Build history of the part. All positions in model axes, mm. A direction names the side the tool comes from. Give positions to 0.01 mm unless a question says otherwise; leave off trailing zeros. Order: outer loops, then holes, each group sorted by start corner. A loop starts at its lowest first (then second) coordinate and runs counter-clockwise, first axis right, second up. Notation, with made-up numbers: M -0.75,48.5 L 39.25,48.5 A16 ccw 39.25,52.5 Z; hole C -29,56 d5. An arc over 180 degrees is marked long. One line per item, written item: value. Start each with the question number.
Autodesk Inventor part; units mm, degrees
ref_plane "YZ Plane" through (0, 0, 0) normal (1, 0, 0) x (0, 1, 0)
ref_plane "XZ Plane" through (0, 0, 0) normal (0, 1, 0) x (-1, 0, 0)
ref_plane "XY Plane" through (0, 0, 0) normal (0, 0, 1) x (1, 0, 0)
sketch "Sketch1" plane through (0, 0, 0) normal (0, 0, 1) x (1, 0, 0)
  line L0 (0, 0) -> (25.4, 0)
  line L1 (25.4, 0) -> (25.4, 25.4)
  line L2 (25.4, 25.4) -> (0, 25.4)
  line L3 (0, 25.4) -> (0, 0)
  line L4 (1.5875, 23.8125) -> (23.8125, 23.8125)
  line L5 (23.8125, 23.8125) -> (23.8125, 1.5875)
  line L6 (23.8125, 1.5875) -> (1.5875, 1.5875)
  line L7 (1.5875, 1.5875) -> (1.5875, 23.8125)
  dimension "d0" = 25.4
  dimension "d1" = 25.4
  dimension "d2" = 1.5875
extrude "Extrusion1" add sketch "Sketch1" against normal blind 330.2
sketch "Sketch2" plane through (0, 0, 0) normal (0, -1, 0) x (1, 0, 0)
  line L0 (0, -330.2) -> (25.4, -330.2)
  point P0 (12.7, -127)
  point P1 (12.7, -88.9)
  dimension "d5" = 38.1
  dimension "d6" = 203.2
hole "Hole1" at (12.7, 0, -127) at (12.7, 0, -88.9) direction (0, 1, 0) diameter 6.35 depth 25.4 tip angle 118
properties part number "1tube_13_layer1_side"
1) Drill centre lines: line 1 (Z direction, x = 12.7, y = 0.7) (3 decimals); line 2 (X direction, y = 24.35, z = -127) (3 decimals); line 3 (X direction, y = 7.75, z = -239.5). Where is each one in solid material? Low to high.
2) Slice it at B-B (x = 12.7). List the corners of the cut face in (y, z) (1 decimal), plus the area to 3 significant figures.
3) Tool access for faces 1 (the cylindrical face through (13.92, 24.62, -129.93)), 2 (the flat face through (23.812, 13, -163)): list every direction of +Z, -Z, +X, -X, +Y, -Y with a clear straight run to the whole face (end or side of a thin tool).
4) Pull direction Y, two halves, no side cores. Call faces 3 (the flat face through (13, 25.4, -163)), 4 (the flat face through (13, 1.588, -163)), 5 (the cylindrical face through (13.92, 0.8, -129.93)): pulls with the +Y half, pulls with the -Y half, needs draft (parallel to the pull), parting line crosses it, or undercut.
5) Slice it at C-C (z = -88.9). List the corners of the cut face in (x, y) (1 decimal).
6) Slice it at A-A (y = 11.5). List the corners of the cut face in (x, z), plus the area to 3 significant figures.
7) Drop flat-ended pins along their axis: P1, Ø4, axis at x = 12.7, z = -127, coming from the -Y side; P2, Ø3, axis at x = 19, z = -166, coming from the -Y side. Give the stop position or say it passes through.
Results list:
1. line 1: z = -330.2 to -130.175, -123.825 to -92.075, -85.725 to 0
1. line 2: x = 0 to 9.525, 15.875 to 25.4
1. line 3: x = 0 to 1.59, 23.81 to 25.4
2. outline: M 0,-330.2 L 1.6,-330.2 L 1.6,-130.2 L 0,-130.2 Z; M 0,-123.8 L 1.6,-123.8 L 1.6,-92.1 L 0,-92.1 Z; M 0,-85.7 L 1.6,-85.7 L 1.6,0 L 0,0 Z; M 23.8,-330.2 L 25.4,-330.2 L 25.4,-130.2 L 23.8,-130.2 Z; M 23.8,-123.8 L 25.4,-123.8 L 25.4,-92.1 L 23.8,-92.1 Z; M 23.8,-85.7 L 25.4,-85.7 L 25.4,0 L 23.8,0 Z
2. area: 1,010 mm²
3. face 1: +Y, -Y
3. face 2: +Z, -Z
4. face 3: pulls with the +Y half
4. face 4: undercut
4. face 5: needs draft
5. outline: M 0,0 L 9.5,0 L 9.5,1.6 L 1.6,1.6 L 1.6,23.8 L 9.5,23.8 L 9.5,25.4 L 0,25.4 Z; M 15.9,0 L 25.4,0 L 25.4,25.4 L 15.9,25.4 L 15.9,23.8 L 23.8,23.8 L 23.8,1.6 L 15.9,1.6 Z
6. outline: M 0,-330.2 L 1.59,-330.2 L 1.59,0 L 0,0 Z; M 23.81,-330.2 L 25.4,-330.2 L 25.4,0 L 23.81,0 Z
6. area: 1,050 mm²
7. P1: passes through
7. P2: stops at y = 0
